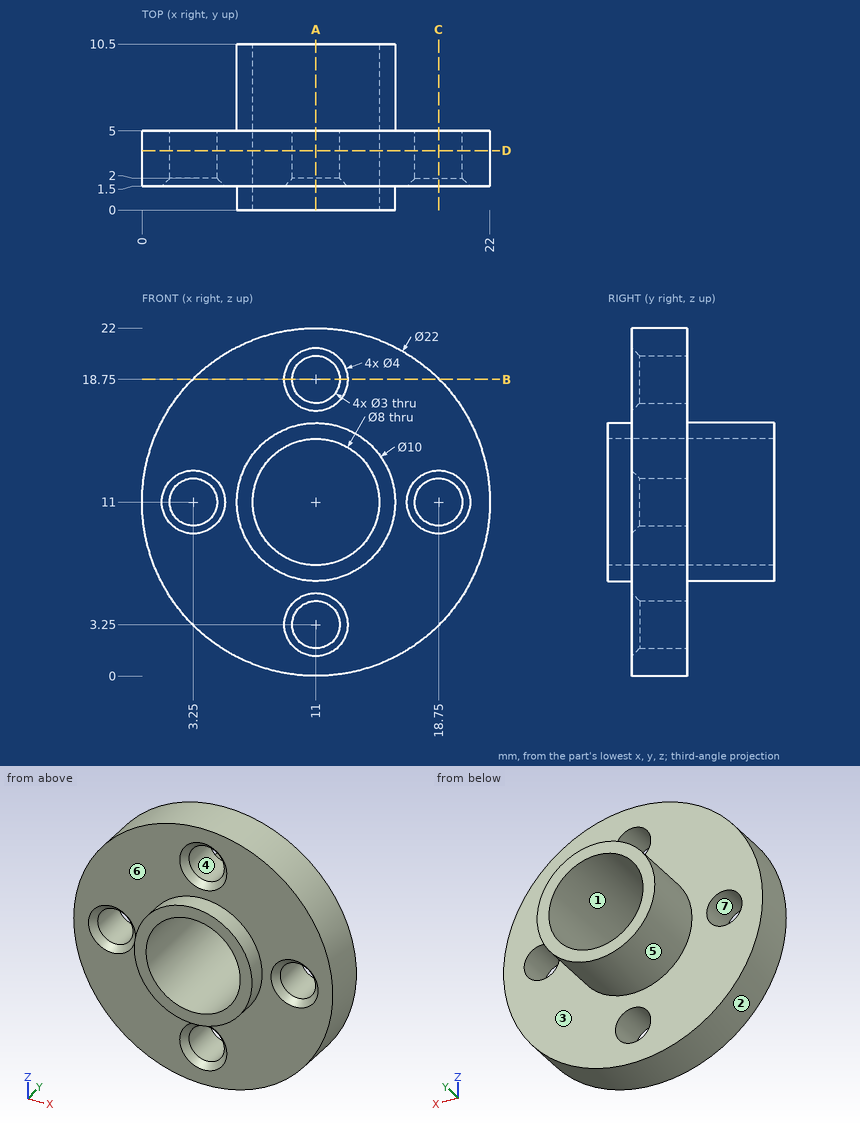
Answer from the drawing. Dimensions are ordinates in mm from the lowest x, y and z of the part. A direction names the side the tool comes from. Give positions to 0.01 mm unless a question says otherwise; leave off trailing zeros. Loops run counter-clockwise (first coordinate to the right, second up) from the corner with the lowest first, then second, coordinate; pieces in that order, holes last.
Item 1: Find the intervals of material crossed by line 1 along Z through (x, y) = (11, 2.5); line 2 along Y through (x, z) = (15, 7.5); line 3 along X through (y, z) = (6.75, 9.5), in increasing order.
Derived:
line 1: z = 0 to 1.75, 4.75 to 7, 15 to 17.25, 20.25 to 22
line 2: y = 1.5 to 5
line 3: x = 6.23 to 7.29, 14.71 to 15.77
Item 2: Each of these flat-tipped pins is pushed along its axis until it touches: pin 1 Ø3 at (x, y) = (4.5, 1.5) entering from -Z; pin 2 Ø1 at (y, z) = (6, 5) entering from -X; pin 3 Ø3.5 at (x, z) = (11, 3.25) entering from -Y; pin 4 Ø4 at (x, z) = (3.25, 11) entering from +Y. Where does it stop, or does it pass through?
Derived:
pin 1: stops at z = 1.2
pin 2: passes through
pin 3: stops at y = 1.75
pin 4: stops at y = 5
Item 3: A cutting plane is placed at A-A (x = 11). Give the vertices of the cut face in (y, z).
Derived:
outline: (0, 6) - (1.5, 6) - (1.5, 5.25) - (2, 4.75) - (5, 4.75) - (5, 6) - (10.5, 6) - (10.5, 7) - (0, 7) - close; (0, 15) - (10.5, 15) - (10.5, 16) - (5, 16) - (5, 17.25) - (2, 17.25) - (1.5, 16.75) - (1.5, 16) - (0, 16) - close; (1.5, 0) - (5, 0) - (5, 1.75) - (2, 1.75) - (1.5, 1.25) - close; (1.5, 20.75) - (2, 20.25) - (5, 20.25) - (5, 22) - (1.5, 22) - close
Item 4: A tool of negligible diameter and unlimited length cuts with its end or side. For the marked faces 5, 6 and 7, from which of +Z, -Z, +X, -X, +Y, -Y can it reach the whole face along a straight path? Write none if from no direction.
Derived:
face 5: +Y
face 6: -Y
face 7: +Y, -Y
Item 5: Determine the mould class of the marked faces 1, 2, 3 and 4 for opening direction Z: +Z half, -Z half, draft (parallel to the pull), parting line (faces both ways), or undercut.
Derived:
face 1: undercut
face 2: parting line
face 3: draft
face 4: undercut
Item 6: A cutting plane is placed at C-C (x = 18.75). Give the vertices of the cut face in (y, z).
Derived:
outline: (1.5, 3.19) - (5, 3.19) - (5, 9.5) - (2, 9.5) - (1.5, 9) - close; (1.5, 13) - (2, 12.5) - (5, 12.5) - (5, 18.81) - (1.5, 18.81) - close
Item 7: A cutting plane is placed at B-B (z = 18.75). Give the vertices of the cut face in (x, y), then the cut area to 3 significant figures.
Derived:
outline: (3.19, 1.5) - (9, 1.5) - (9.5, 2) - (9.5, 5) - (3.19, 5) - close; (12.5, 2) - (13, 1.5) - (18.81, 1.5) - (18.81, 5) - (12.5, 5) - close
area: 43.9 mm2
Item 8: A cutting plane is placed at D-D (y = 3.75). Give the vertices of the cut face in (x, z), then the cut area to 3 significant figures.
Derived:
outline: circle Ø22 at (11, 11); hole circle Ø3 at (3.25, 11); hole circle Ø8 at (11, 11); hole circle Ø3 at (11, 3.25); hole circle Ø3 at (11, 18.75); hole circle Ø3 at (18.75, 11)
area: 302 mm2
